Here's how the part is built. I have some questions about the finished solid (model axes, mm). Give positions to 0.01 mm unless a question says otherwise; leave off trailing zeros. Write each loop counter-clockwise with the first axis right and the second up, starting at its lowest first coordinate (ties: lowest second). Pieces come first, ordered by that corner, then holes. Notation, with made-up numbers: M 42.5,65.25 L 75.5,65.25 A21 ccw 75.5,103.25 Z; hole C 56,64.25 d2. An arc over 180 degrees is marked long. Use one line per item in the form item = value. Start each with the question number.
from build123d import *

# Parameters (mm, degrees)
F0_R     = 2.5
F1_DEPTH = 5
F2_R     = 2.5
F3_DEPTH = 120


with BuildPart() as f1:
    # F0 (on Front) → F1 (new body, symmetric)
    with BuildSketch(Plane.XZ):
        with BuildLine():
            Line((-55, -10), (55, -10))
            ThreePointArc((55, -10), (58.535534, -8.535534), (60, -5))
            Line((60, -5), (60, 5))
            ThreePointArc((60, 5), (58.535534, 8.535534), (55, 10))
            Line((55, 10), (-55, 10))
            ThreePointArc((-55, 10), (-58.535534, 8.535534), (-60, 5))
            Line((-60, 5), (-60, -5))
            ThreePointArc((-60, -5), (-58.535534, -8.535534), (-55, -10))
        make_face()
        with Locations((-50, 0)):
            Circle(F0_R, mode=Mode.SUBTRACT)
        with Locations((-25, 0)):
            Circle(F0_R, mode=Mode.SUBTRACT)
        with BuildLine():
            ThreePointArc((47.5, 0), (50, 2.5), (52.5, 0))
            ThreePointArc((52.5, 0), (50, -2.5), (47.5, 0))
        make_face(mode=Mode.SUBTRACT)
    extrude(amount=F1_DEPTH, both=True)

    # F2 (on face) → F3 (cut)
    with BuildSketch(Plane(origin=(-60, 0, 0), x_dir=(0, -1, 0), z_dir=(-1, 0, 0))):
        Circle(F2_R)
    extrude(amount=-F3_DEPTH, mode=Mode.SUBTRACT)


solid = f1.part
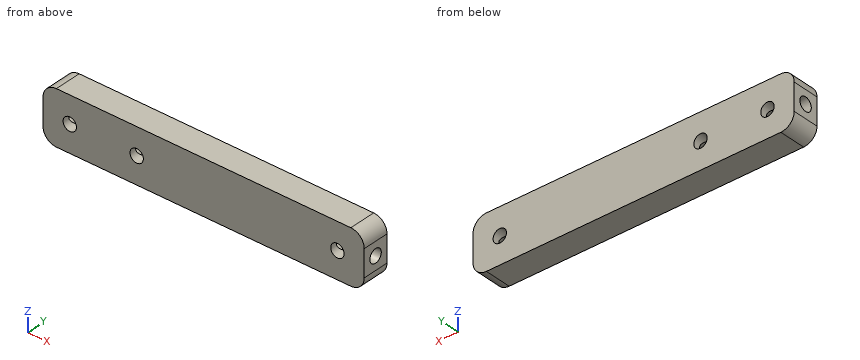
1) Suppose I cut it at B-B, the plane x = -17. List the corners of the cut face in (y, z) for me.
2) Will this pin go through, and if not, where does the flat tip stop? P1, Ø3, axis at y = -3, z = -7, coming from the -X side.
3) Suppose I cut it at A-A, the plane y = -4. List the corners of the cut face in (x, z) for me, and give its area (3 significant figures).
4) Suppose I cut it at C-C, the plane z = 0. State how many separate pieces and enclosed holes the cut face has, and give its area (3 significant figures).
5) Please list where these lines run through material, in increasing order: line 1 (X direction, y = 4.25, z = -0.25); line 2 (Y direction, x = -0.5, z = 0); line 3 (X direction, y = 2.75, z = 2).
Checks:
q1.outline = M -5,-10 L 5,-10 L 5,10 L -5,10 Z; hole C 0,0 d5
q2.P1 = -59.97
q3.outline = M -60,-5 A5 ccw -55,-10 L 55,-10 A5 ccw 60,-5 L 60,5 A5 ccw 55,10 L -55,10 A5 ccw -60,5 Z; hole C -50,0 d5; hole C -25,0 d5; hole C 50,0 d5
q3.area = 2,320 mm^2
q4.separate_pieces = 8
q4.enclosed_holes = 0
q4.area = 525 mm^2
q5.line_1 = -60 to -52.49, -47.51 to -27.49, -22.51 to 47.51, 52.49 to 60
q5.line_2 = -5 to -2.5, 2.5 to 5
q5.line_3 = -60 to -51.5, -48.5 to -26.5, -23.5 to 48.5, 51.5 to 60
